Autodesk Inventor part; units mm, degrees
ref_plane "YZ Plane" through (0, 0, 0) normal (1, 0, 0) x (0, 1, 0)
ref_plane "XZ Plane" through (0, 0, 0) normal (0, 1, 0) x (-1, 0, 0)
ref_plane "XY Plane" through (0, 0, 0) normal (0, 0, 1) x (1, 0, 0)
sketch "Sketch1" plane through (0, 0, 0) normal (1, 0, 0) x (0, 1, 0)
  line L0 (0, 0) -> (25.4, 0)
  line L1 (0, 0) -> (0, -25.4)
  line L2 (0, -25.4) -> (3.175, -25.4)
  line L3 (25.4, 0) -> (25.4, -3.175)
  line L4 (25.4, -3.175) -> (3.175, -3.175)
  line L5 (3.175, -3.175) -> (3.175, -25.4)
  dimension "d0" = 25.4
  dimension "d1" = 25.4
  dimension "d2" = 3.175
  dimension "d3" = 3.175
extrude "Extrusion1" add sketch "Sketch1" along normal mid plane 25.4
sketch "Sketch2" plane through (-12.7, 3.175, -3.175) normal (0, 1, 0) x (1, 0, 0)
  line L0 (0, 0) -> (25.4, 0) construction
  line L1 (25.4, 22.225) -> (25.4, 0) construction
  line L2 (25.4, 22.225) -> (0, 22.225) construction
  line L3 (0, 0) -> (0, 22.225) construction
  line L4 (12.7, 22.225) -> (12.7, 0) construction
  line L5 (0, 11.1125) -> (25.4, 11.1125) construction
  circle A0 centre (18.7, 17.1125) radius 2
  circle A1 centre (6.7, 17.1125) radius 2
  circle A2 centre (6.7, 5.1125) radius 2
  circle A3 centre (18.7, 5.1125) radius 2
  point P0 (12.7, -3.175)
  point P1 (12.7, 11.1125)
  point P2 (12.7, 11.1125)
  dimension "d7" = 4
  dimension "d8" = 6
  dimension "d32" = 6
  dimension "d35" = 360
extrude "Extrusion2" cut sketch "Sketch2" against normal through all contours A0
sketch "Sketch3" plane through (12.7, 25.4, -3.175) normal (0, 0, -1) x (-1, 0, 0)
  line L0 (25.4, 0) -> (0, 0) construction
  line L1 (0, -22.225) -> (0, 0) construction
  line L2 (25.4, -22.225) -> (0, -22.225) construction
  line L3 (25.4, 0) -> (25.4, -22.225) construction
  line L4 (12.7, 0) -> (12.7, -22.225) construction
  line L5 (0, -11.1125) -> (25.4, -11.1125) construction
  circle A0 centre (18.7, -5.1125) radius 2
  circle A1 centre (6.7, -5.1125) radius 2
  circle A2 centre (6.7, -17.1125) radius 2
  circle A3 centre (18.7, -17.1125) radius 2
  point P0 (12.7, -25.4)
  point P1 (12.7, -11.1125)
  point P2 (12.7, -11.1125)
  dimension "d13" = 4
  dimension "d14" = 6
  dimension "d39" = 6
  dimension "d42" = 360
extrude "Extrusion3" cut sketch "Sketch3" against normal through all contours A0
extrude "Extrusion4" cut sketch "Sketch2" against normal through all contours A1 | A2 | A3
extrude "Extrusion5" cut sketch "Sketch3" against normal through all contours A1 | A2 | A3
hole "Hole3" at (6, 3.175, -8.2875) at (-6, 3.175, -8.2875) at (-6, 3.175, -20.2875) at (6, 3.175, -20.2875) direction (0, -1, 0) diameter 4 end through all countersink diameter 8 countersink angle 90
hole "Hole4" at (6, 8.2875, -3.175) at (-6, 8.2875, -3.175) at (-6, 20.2875, -3.175) at (6, 20.2875, -3.175) direction (0, 0, 1) diameter 4 end through all countersink diameter 8 countersink angle 90
properties part number "Arashtrix 1in x 1in L-Bracket"
Part model, mm, in its own coordinate system. A direction names the side the tool comes from. Give positions to 0.01 mm unless a question says otherwise; leave off trailing zeros. Loops run counter-clockwise (first coordinate to the right, second up) from the corner with the lowest first, then second, coordinate; pieces in that order, holes last. Notation, with made-up numbers: M 60,35 L 90,35 A26 cw 90,63 Z; hole C 30,4.5 d2. An arc over 180 degrees is marked long. Put each result on its own line as item: value. Start each with the question number.
1) Pull direction X, two halves, no side cores. Call faces 1 (the conical face through (-6.81, 1.3, -18.32)), 2 (the conical face through (8.107, 20.011, -1.3)), 3 (the flat face through (12.7, 2, -7)), 4 (the flat face through (0, 25.4, -2)): +X half, -X half, draft (parallel to the pull), parting line (faces both ways), or undercut.
2) Probe probe 1 along Y at (x, z) = (6, -0.45); probe 2 along Z at (x, y) = (6, 0.8); probe 3 along X at (y, z) = (2, -20.25). List the from-to ranges inside material, lowest first.
3) Saw through at B-B (x = -1.5). List the corners of the cut face in (y, z) (3 decimals).
4) Saw through at A-A (x = 6). State how many separate pieces and enclosed holes the cut face has, then the cut area to 3 significant figures.
5) Saw through at C-C (y = 14.25). List the corners of the cut face in (x, z) (3 decimals), then the cut area to 3 significant figures.
6) Flat gauge pins, fed straight in: pin 1 (6 mm diameter, centred on y = 19, z = -3.5, fed in from -X); pin 2 (4.5 mm diameter, centred on x = -6, y = 20.29, fed in from -Z); pin 3 (6.5 mm diameter, centred on x = 6, y = 8.29, fed in from -Z); pin 4 (1.5 mm diameter, centred on x = -10, z = -18, fed in from +Y) (3 decimals). Where does each tip first touch, or does it go through?
7) 3-axis set-ups, long thin cutter, end or side, ignore diameter. For faces 5 (the flat face through (-12.7, 2, -7)), 6 (the flat face through (0, 3.175, -14)): which of +Z, -Z, +X, -X, +Y, -Y reach the whole face in a straight line?
Numbers:
1. face 1: undercut
1. face 2: undercut
1. face 3: +X half
1. face 4: draft
2. probe 1: 0 to 6.29, 10.29 to 18.29, 22.29 to 25.4
2. probe 2: -25.4 to -22.29, -18.29 to -10.29, -6.29 to 0
2. probe 3: -12.7 to -8.82, -3.18 to 3.18, 8.82 to 12.7
3. outline: M 0,-25.4 L 3.175,-25.4 L 3.175,-3.175 L 25.4,-3.175 L 25.4,0 L 0,0 Z
4. separate pieces: 5
4. enclosed holes: 0
4. area: 84.4 mm^2
5. outline: M -12.7,-3.175 L 12.7,-3.175 L 12.7,0 L -12.7,0 Z
5. area: 80.6 mm^2
6. pin 1: x = -12.7
6. pin 2: z = -1.43
6. pin 3: z = -2.43
6. pin 4: y = 3.175
7. face 5: +Z, -Z, -X, +Y, -Y
7. face 6: -Z, +X, -X, +Y
